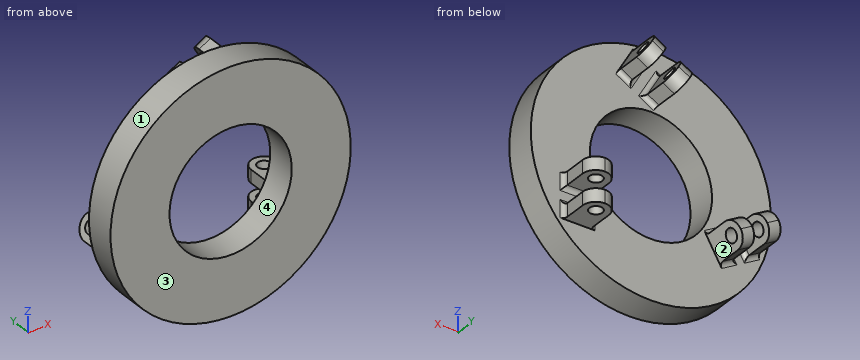
```python
from build123d import *

# Parameters (mm, degrees)
SKETCH1_R                = 27.5
SKETCH1_R_2              = 14
BOSS_EXTRUDE1_DEPTH      = 7
SKETCH3_W                = 6
SKETCH3_H                = 3
BOSS_EXTRUDE2_DEPTH      = 9
FILLET1_R                = 3
FILLET2_R                = 1
SKETCH5_R                = 1.5
CUT_EXTRUDE2_DEPTH       = 47.703277471
CIRPATTERN2_COUNT        = 3
FILLET1_OF_CIRPATTERN2_R = 3
FILLET2_OF_CIRPATTERN2_R = 1


with BuildPart() as part:
    # Sketch1 → Boss-Extrude1 (new body)
    with BuildSketch(Plane(origin=(0, 0, 0), x_dir=(1, 0, 0), z_dir=(0, 1, 0))):
        with Locations(Location((0, 0, 0), (0, 0, 270))):
            Circle(SKETCH1_R)
        with Locations(Location((0, 0, 0), (0, 0, 270))):
            Circle(SKETCH1_R_2, mode=Mode.SUBTRACT)
    extrude(amount=BOSS_EXTRUDE1_DEPTH)

    # Sketch3 → Boss-Extrude2 (add)
    with BuildSketch(Plane(origin=(0, 7, 0), x_dir=(1, 0, 0), z_dir=(0, 1, 0))):
        with Locations((16.852148123, 8.189854147)):
            Rectangle(SKETCH3_W, SKETCH3_H)
        with Locations((16.852148123, 15.189854147)):
            Rectangle(SKETCH3_W, SKETCH3_H)
    boss_extrude2 = extrude(amount=BOSS_EXTRUDE2_DEPTH)

    # Fillet1
    fillet1_edges = [part.edges().sort_by_distance(p)[0] for p in [
        (19.852148123, 16, -8.189854147),
        (13.852148123, 16, -8.189854147),
        (13.852148123, 16, -15.189854147),
        (19.852148123, 16, -15.189854147),
    ]]
    fillet(fillet1_edges, radius=FILLET1_R - 0.0001)  # a hair under: the kernel refuses the full size

    # Fillet2
    fillet2_edges = [part.edges().sort_by_distance(p)[0] for p in [
        (19.852148123, 7, -8.189854147),
        (16.852148123, 7, -9.689854147),
        (13.852148123, 7, -8.189854147),
        (19.852148123, 7, -15.189854147),
        (13.852148123, 7, -15.189854147),
        (16.852148123, 7, -13.689854147),
    ]]
    fillet(fillet2_edges, radius=FILLET2_R)

    # Sketch5 → Cut-Extrude2 (cut, symmetric)
    with BuildSketch(Plane.XY.offset(-6.689854147)):
        with Locations((16.823138997, 13)):
            Circle(SKETCH5_R)
    cut_extrude2 = extrude(amount=CUT_EXTRUDE2_DEPTH, both=True, mode=Mode.SUBTRACT)

    # CirPattern2: Boss-Extrude2, Cut-Extrude2 ×3 about axis
    cirpattern2_axis = Axis((0, 0, 0), (0, 1, 0))
    add([boss_extrude2.rotate(cirpattern2_axis, i * 360 / CIRPATTERN2_COUNT) for i in range(1, CIRPATTERN2_COUNT)])
    add([cut_extrude2.rotate(cirpattern2_axis, i * 360 / CIRPATTERN2_COUNT) for i in range(1, CIRPATTERN2_COUNT)], mode=Mode.SUBTRACT)

    # Fillet1 of CirPattern2
    fillet1_of_cirpattern2_edges = [part.edges().sort_by_distance(p)[0] for p in [
        (-17.018695806, 16, -13.097537521),
        (-14.018695806, 16, -7.901385098),
        (-20.080873632, 16, -4.401385098),
        (-23.080873632, 16, -9.597537521),
        (-2.833452317, 16, 21.287391668),
        (0.166547683, 16, 16.091239245),
        (6.228725509, 16, 19.591239245),
        (3.228725509, 16, 24.787391668),
    ]]
    fillet(fillet1_of_cirpattern2_edges, radius=FILLET1_OF_CIRPATTERN2_R - 0.0001)  # a hair under: the kernel refuses the full size

    # Fillet2 of CirPattern2
    fillet2_of_cirpattern2_edges = [part.edges().sort_by_distance(p)[0] for p in [
        (-17.018695806, 7, -13.097537521),
        (-16.817733912, 7, -9.749461309),
        (-14.018695806, 7, -7.901385098),
        (-23.080873632, 7, -9.597537521),
        (-20.080873632, 7, -4.401385098),
        (-20.281835527, 7, -7.749461309),
        (-2.833452317, 7, 21.287391668),
        (-0.034414211, 7, 19.439315456),
        (0.166547683, 7, 16.091239245),
        (3.228725509, 7, 24.787391668),
        (6.228725509, 7, 19.591239245),
        (3.429687404, 7, 21.439315456),
    ]]
    fillet(fillet2_of_cirpattern2_edges, radius=FILLET2_OF_CIRPATTERN2_R)


solid = part.part
```
Input: part model. Units: mm. Frame: model coordinates. Face numbers are marked on the shaded views. Coordinates: 2 decimals unless noted, no trailing zeros. Write each loop counter-clockwise with the first axis right and the second up, starting at its lowest first coordinate (ties: lowest second). Pieces come first, ordered by that corner, then holes. Notation, with made-up numbers: M -4.75,-11 L 49.25,-11 A26 cw 49.25,10 Z; hole C 88.5,1 d7. An arc over 180 degrees is marked long. Use one line per item in the form item = value.
Q1. Section A-A (z = 0). Return loops of the section in (x, y), plus the area to 3 significant figures.
Answer below:
outline = M -27.5,0 L -14,0 L -14,7 L -27.5,7 Z; M 14,0 L 27.5,0 L 27.5,7 L 14,7 Z
area = 189 mm²
Q2. Section B-B (y = 6). Return loops of the section in (x, z), plus the area to 3 significant figures.
Answer below:
outline = C 0,0 d55; hole C 0,0 d28
area = 1,760 mm²
Q3. Material intervals for probe 1 along X at (y, z) = (4, 0); probe 2 along X at (y, z) = (8.5, -10); probe 3 along Y at (x, z) = (15.5, -7.5), sorted ascending. Write a range as from..to.
Answer below:
probe_1 = -27.5..-14, 14..27.5
probe_2 = -22.38..-21.58, -16.96..-13.5
probe_3 = 0..12.29, 13.71..15.68
Q4. Draft query along Z for the marked faces 1, 2, 3 and 4. Return one class per face: released by +Z, released by -Z, zero draft, split by the parting line, or undercut.
Answer below:
face_1 = split by the parting line
face_2 = released by -Z
face_3 = zero draft
face_4 = undercut
Q5. First-contact query: pin 1 (2 mm diameter, centred on x = -3, z = 11, fed in from -Y); pin 2 (8 mm diameter, centred on x = 22, z = -16, fed in from -Y); pin 3 (0.9 mm diameter, centred on y = 9.5, z = -14.5, fed in from +X); pin 4 (3 mm diameter, centred on x = 3.5, z = -18.5, fed in from +Y). Flat tips, straight axial feed; report the tip coordinate or a pass-through.
Answer below:
pin_1 = through
pin_2 = 0
pin_3 = 19.85
pin_4 = 7
